Could you check a few things on this model? Use its own coordinates, in mm. Round coordinates to 2 decimals unless told otherwise and drop trailing zeros. Loops run counter-clockwise (first coordinate to the right, second up) from the corner with the lowest first, then second, coordinate; pieces in that order, holes last.
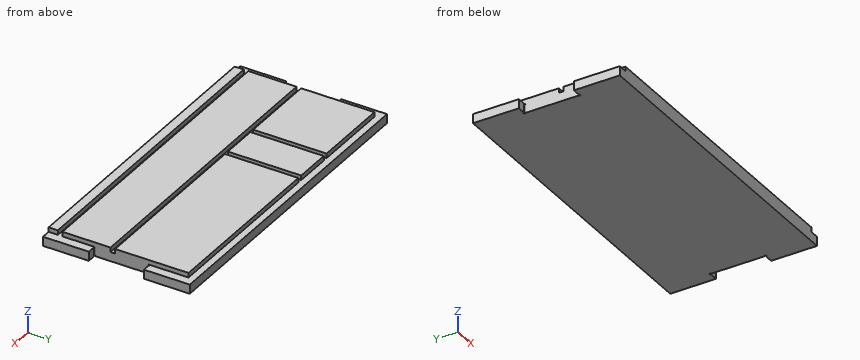
from build123d import *

# Parameters (mm, degrees)
F0_W     = 222.25
F0_H     = 101.6
F1_DEPTH = 9.525
F2_W     = 6.35
F2_H     = 38.1
F3_DEPTH = 9.526
F4_W     = 6.35
F4_H     = 31.75
F5_DEPTH = 3.175
F6_W     = 209.55
F6_H     = 3.175
F6_W_2   = 3.175
F6_H_2   = 50.8
F7_DEPTH = 3.175
F9_DEPTH = 6.35


with BuildPart() as f1:
    # F0 (on Top) → F1 (new body)
    with BuildSketch(Plane.XY):
        Rectangle(F0_W, F0_H)
    extrude(amount=F1_DEPTH)

    # F2 (on face) → F3 (cut, through all)
    with BuildSketch(Plane.XY.offset(9.525)):
        with Locations((-107.95, 0)):
            Rectangle(F2_W, F2_H)
        with Locations((107.95, 0)):
            Rectangle(F2_W, F2_H)
    extrude(amount=-F3_DEPTH, mode=Mode.SUBTRACT)

    # F4 (on face) → F5 (cut)
    with BuildSketch(Plane.XY.offset(9.525)):
        Polygon((-111.125, 19.05), (-104.775, 19.05), (-104.775, 46.0248), (104.775, 46.0248), (104.775, 19.05), (111.125, 19.05), (111.125, 50.8), (-111.125, 50.8), align=None)
        with Locations((-107.95, -34.925)):
            Rectangle(F4_W, F4_H)
        with Locations((107.95, -34.925)):
            Rectangle(F4_W, F4_H)
    extrude(amount=-F5_DEPTH, mode=Mode.SUBTRACT)

    # F6 (on face) → F7 (cut)
    with BuildSketch(Plane.XY.offset(9.525)):
        with Locations((0, -42.8625)):
            Rectangle(F6_W, F6_H)
        Polygon((-50.8, -4.7752), (-104.775, -4.7752), (-104.775, -7.9502), (104.775, -7.9502), (104.775, -4.7752), (-19.05, -4.7752), (-22.225, -4.7752), (-47.625, -4.7752), align=None)
        with Locations((-49.2125, 20.6248)):
            Rectangle(F6_W_2, F6_H_2)
        with Locations((-20.6375, 20.6248)):
            Rectangle(F6_W_2, F6_H_2)
    extrude(amount=-F7_DEPTH, mode=Mode.SUBTRACT)

    # F8 (on face) → F9 (cut, through all)
    with BuildSketch(Plane(origin=(0, 0, 0), x_dir=(1, 0, 0), z_dir=(0, 0, -1))):
        with BuildLine():
            Line((104.775, -19.05), (104.775, -18.415))
            ThreePointArc((104.775, -18.415), (104.325987, -19.499013), (105.41, -19.05))
            Line((105.41, -19.05), (104.775, -19.05))
        make_face()
        with BuildLine():
            ThreePointArc((105.41, 19.05), (104.325987, 19.499013), (104.775, 18.415))
            Line((104.775, 18.415), (104.775, 19.05))
            Line((104.775, 19.05), (105.41, 19.05))
        make_face()
        with BuildLine():
            Line((-104.775, 19.05), (-104.775, 18.415))
            ThreePointArc((-104.775, 18.415), (-104.325987, 19.499013), (-105.41, 19.05))
            Line((-105.41, 19.05), (-104.775, 19.05))
        make_face()
        with BuildLine():
            ThreePointArc((-105.41, -19.05), (-104.325987, -19.499013), (-104.775, -18.415))
            Line((-104.775, -18.415), (-104.775, -19.05))
            Line((-104.775, -19.05), (-105.41, -19.05))
        make_face()
    extrude(amount=-F9_DEPTH, mode=Mode.SUBTRACT)


solid = f1.part
Item 1: If we section it at D-D, the plane y = -12: Please give me the cut outline in (x, z) (3 decimals), then the cut area to 3 significant figures.
Results list:
outline: (-104.775, 0) - (104.775, 0) - (104.775, 9.525) - (-104.775, 9.525) - close
area: 2,000 mm2
Item 2: If we section it at B-B, the plane y = 0: Please give me the cut outline in (x, z) (3 decimals).
Results list:
outline: (-104.775, 0) - (104.775, 0) - (104.775, 9.525) - (-19.05, 9.525) - (-19.05, 6.35) - (-22.225, 6.35) - (-22.225, 9.525) - (-47.625, 9.525) - (-47.625, 6.35) - (-50.8, 6.35) - (-50.8, 9.525) - (-104.775, 9.525) - close
Item 3: If we section it at C-C, the plane z = 3.25: Please give me the cut outline in (x, y) (3 decimals), then the cut area to 3 significant figures.
Results list:
outline: (-111.125, -50.8) - (111.125, -50.8) - (111.125, -19.05) - (105.41, -19.05) arc R0.635 cw (long way) to (104.775, -18.415) - (104.775, 18.415) arc R0.635 cw (long way) to (105.41, 19.05) - (111.125, 19.05) - (111.125, 50.8) - (-111.125, 50.8) - (-111.125, 19.05) - (-105.41, 19.05) arc R0.635 cw (long way) to (-104.775, 18.415) - (-104.775, -18.415) arc R0.635 cw (long way) to (-105.41, -19.05) - (-111.125, -19.05) - close
area: 22,100 mm2
Item 4: If we section it at A-A, the plane x = 81.5: Please give me the cut outline in (y, z) (3 decimals), then the cut area to 3 significant figures.
Results list:
outline: (-50.8, 0) - (50.8, 0) - (50.8, 6.35) - (46.025, 6.35) - (46.025, 9.525) - (-4.775, 9.525) - (-4.775, 6.35) - (-7.95, 6.35) - (-7.95, 9.525) - (-41.275, 9.525) - (-41.275, 6.35) - (-44.45, 6.35) - (-44.45, 9.525) - (-50.8, 9.525) - close
area: 932 mm2
Item 5: If I drill on line 1 along Y through (x, z) = (23, 8.5) (3 decimals); line 2 along X through (y, z) = (7.5, 9.25) (3 decimals); line 3 along X through (y, z) = (-16, 2.5) (3 decimals), over which ranges is the centre line in solid material (lowest first)?
Results list:
line 1: y = -50.8 to -44.45, -41.275 to -7.95, -4.775 to 46.025
line 2: x = -104.775 to -50.8, -47.625 to -22.225, -19.05 to 104.775
line 3: x = -104.775 to 104.775
Item 6: Will these pins go through, and if not, where does the flat tip stop? pin 1 (1.6 mm diameter, centred on x = -34.5, z = 7, fed in from +Y); pin 2 (1 mm diameter, centred on x = -70.5, z = 8, fed in from +Y); pin 3 (1 mm diameter, centred on y = 18, z = 8.5, fed in from -X) (3 decimals); pin 4 (1 mm diameter, centred on y = 32.5, z = 7.5, fed in from +X) (3 decimals).
Results list:
pin 1: stops at y = 50.8
pin 2: stops at y = 46.02
pin 3: stops at x = -104.775
pin 4: stops at x = 104.775
